Check sheet for the modelled part. Datum: model origin and axes. Units: mm. Face numbers are marked on the shaded views. Give positions to 0.01 mm unless a question says otherwise; leave off trailing zeros. Order: outer loops, then holes, each group sorted by start corner. A loop starts at its lowest first (then second) coordinate and runs counter-clockwise, first axis right, second up.
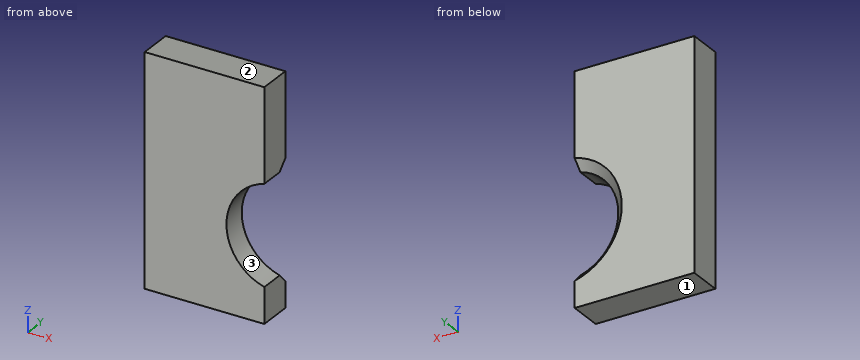
```python
from build123d import *

# Parameters (mm, degrees)
BOSS_EXTRUDE1_DEPTH = 3.7
CHAMFER1_SIZE       = 1


with BuildPart() as part:
    # Sketch1 → Boss-Extrude1 (new body)
    with BuildSketch(Plane(origin=(0, 0, 0), x_dir=(1, 0, 0), z_dir=(0, 1, 0))):
        with BuildLine():
            Line((0, 28.997247011), (0, 4))
            Line((0, 4), (13.1, 4))
            Line((13.1, 4), (13.1, 14.202752989))
            ThreePointArc((13.1, 14.202752989), (8.95, 19.65), (13.1, 25.097247011))
            Line((13.1, 25.097247011), (13.1, 28.997247011))
            Line((13.1, 28.997247011), (0, 28.997247011))
        make_face()
    extrude(amount=BOSS_EXTRUDE1_DEPTH)

    # Chamfer1
    chamfer1_edges = [part.edges().sort_by_distance(p)[0] for p in [
        (8.95, 3.7, -19.65),
    ]]
    chamfer(chamfer1_edges, length=CHAMFER1_SIZE)


solid = part.part
```
(1) Material ranges on L1, parallel to Z at x = 10, y = 1; L2, parallel to Z at x = 10.5, y = 3.55; L3, parallel to X at y = 1.3, z = -19.5, recorded low to high.
Response values:
L1: z = -29 to -22.93, -16.37 to -4
L2: z = -29 to -24.69, -14.61 to -4
L3: x = 0 to 8.95
(2) Release check for a two-part mould opening along Z. For the marked faces 1, 2 and 3 record: released by +Z, released by -Z, zero draft, split by the parting line, or undercut.
Response values:
face 1: released by -Z
face 2: released by +Z
face 3: undercut
(3) Cross-section at A-A on y = 1.1. Enter the section's corners in (x, z), then the cut area to 3 significant figures.
Response values:
outline: (0, -29) - (13.1, -29) - (13.1, -25.1) arc R5.65 cw to (13.1, -14.2) - (13.1, -4) - (0, -4) - close
area: 294 mm2
